Autodesk Inventor part; units mm, degrees
ref_plane "Work Plane2" through (0, 19.05, 0) normal (0, 1, 0) x (1, 0, 0)
ref_plane "YZ Plane" through (0, 0, 0) normal (1, 0, 0) x (0, 1, 0)
ref_plane "XZ Plane" through (0, 0, 0) normal (0, 1, 0) x (-1, 0, 0)
sketch "Sketch1" plane through (0, 0, 0) normal (0, 1, 0) x (-1, 0, 0)
  line L0 (-3.711, -25.8637) -> (-3.711, -32.2137)
  line L1 (-3.711, -32.2137) -> (-49.431, -32.2137)
  line L2 (-49.431, -32.2137) -> (-49.431, -25.8637)
  line L3 (-3.711, -25.8637) -> (-26.571, -6.8137)
  line L4 (-26.571, -6.8137) -> (-49.431, -25.8637)
  point P0 (0, 0)
  dimension "d0" = 6.35
  dimension "d1" = 6.35
  dimension "d2" = 45.72
  dimension "d3" = 22.86
  dimension "d4" = 22.86
  dimension "d5" = 25.4
ref_plane "Work Plane2" through (0, 19.05, 0) normal (0, 1, 0) x (1, 0, 0)
sketch "Sketch2" plane through (0, 19.05, 0) normal (0, 1, 0) x (1, 0, 0)
  line L0 (41.811, 32.2137) -> (11.331, 32.2137)
  line L1 (11.331, 32.2137) -> (11.331, 25.8637)
  line L2 (11.331, 25.8637) -> (26.571, 13.1637)
  line L3 (26.571, 13.1637) -> (41.811, 25.8637)
  line L4 (41.811, 25.8637) -> (41.811, 32.2137)
  point P0 (0, 0)
  point P1 (26.571, 6.8137)
  dimension "d8" = 6.35
  dimension "d9" = 6.35
  dimension "d10" = 15.24
  dimension "d11" = 15.24
  dimension "d12" = 30.48
  dimension "d15" = 0
loft "Loft1" add profiles "Sketch1", "Sketch2"
shell "Shell1" thickness 2.54 removed faces 1 at (26.571, 0, -23.7471)
sketch "Sketch4" plane through (26.571, 0, -6.8137) normal (0.6201737, 0.2480695, 0.7442084) x (0.7682213, 0, -0.6401844)
  line L0 (0, 0) -> (4.0652, 19.6647)
  line L1 (29.7571, 0) -> (23.9032, 19.6647)
  line L2 (29.7571, 0) -> (0, 0)
  line L3 (23.9032, 19.6647) -> (4.0652, 19.6647)
  line L4 (3.1188, 2.54) -> (6.1338, 17.1247)
  line L5 (6.1338, 17.1247) -> (22.0092, 17.1247)
  line L6 (22.0092, 17.1247) -> (26.3508, 2.54)
  line L7 (26.3508, 2.54) -> (3.1188, 2.54)
  point P0 (-24.7744, 2.9212)
  dimension "d21" = 2.54
  dimension "d22" = 2.54
  dimension "d23" = 2.54
  dimension "d24" = 2.54
extrude "Extrusion2" cut sketch "Sketch4" against normal blind 1.27 contours L4 L5 L6 L7
sketch "Sketch5" plane through (3.711, 0, -25.8637) normal (-0.6201737, 0.2480695, 0.7442084) x (0.7682213, 0, 0.6401844)
  line L0 (29.7571, 0) -> (0, 0)
  line L1 (24.1888, 19.6583) -> (4.3507, 19.6583)
  line L2 (3.4063, 2.54) -> (7.746, 17.1183)
  line L3 (7.746, 17.1183) -> (23.6246, 17.1183)
  line L4 (23.6246, 17.1183) -> (26.6383, 2.54)
  line L5 (26.6383, 2.54) -> (3.4063, 2.54)
  line L6 (0, 0) -> (5.8538, 19.6647)
  line L7 (29.7571, 0) -> (25.6919, 19.6647)
  point P0 (13.7067, -5.5182)
  point P1 (-24.7744, 2.9212)
  dimension "d27" = 2.54
  dimension "d29" = 2.54
  dimension "d32" = 2.54
  dimension "d34" = 2.54
extrude "Extrusion3" cut sketch "Sketch5" against normal blind 1.27
sketch "Sketch6" plane through (49.431, 0, -32.2137) normal (0, 0, -1) x (-1, 0, 0)
  circle A0 centre (6.985, 3.175) radius 1.5875
  circle A1 centre (22.86, 15.875) radius 1.5875
  circle A2 centre (38.735, 3.175) radius 1.5875
  line L0 (0, 0) -> (7.62, 19.05)
  line L1 (45.72, 0) -> (0, 0)
  line L2 (45.72, 0) -> (38.1, 19.05)
  line L3 (38.1, 19.05) -> (7.62, 19.05)
  point P0 (49.431, 0)
  dimension "d37" = 6.985
  dimension "d38" = 6.985
  dimension "d39" = 3.175
  dimension "d40" = 3.175
  dimension "d41" = 3.175
  dimension "d42" = 22.86
  dimension "d43" = 3.175
  dimension "d44" = 3.175
  dimension "d45" = 3.175
extrude "Extrusion4" add sketch "Sketch6" along normal blind 3.175 contours A0 | A1 | A2
chamfer "Chamfer1" distance 0.254 angle 45 3 edges at (44.0335, 3.175, -35.3887) (28.1585, 15.875, -35.3887) (12.2835, 3.175, -35.3887)
properties part number "Cow Catcher"
CAD build for the part. Positions are in the model's coordinates, mm. A direction names the side the tool comes from. Round coordinates to 2 decimals unless told otherwise and drop trailing zeros. Order: outer loops, then holes, each group sorted by start corner. A loop starts at its lowest first (then second) coordinate and runs counter-clockwise, first axis right, second up.
Q1. Slice it at A-A (z = -31.75). Write the cut outline in (x, y).
Q2. Which spindle directions (+Z, -Z, +X, -X, +Y, -Y) get a long thin tool onto all of the face, cutting with end or side? Do faces 4 (the cylindrical face through (11.956, 4.141, -33.654)), 5 (the flat face through (35.63, 8.17, -20.5)), 6 (the flat face through (11, 3, -35.389)). Say none if no direction does.
Q3. Drop flat-ended pins along their axis: pin 1 (1 mm diameter, centred on x = 38.5, y = 11, fed in from -Z); pin 2 (6 mm diameter, centred on y = 9, z = -24, fed in from -X); pin 3 (4 mm diameter, centred on x = 36.5, y = 7.5, fed in from +Z); pin 4 (11 mm diameter, centred on x = 33, z = -20, fed in from -Y). Give the stop position or say it passes through.
Q4. Two-plate mould, pull along Y, no slides. Class faces 1 (the flat face through (27, 16, -35.389)), 2 (the flat face through (43.16, 9.47, -24.63)), 3 (the flat face through (45.568, 9.658, -28.994)): pulls with the +Y half, pulls with the -Y half, needs draft (parallel to the pull), parting line crosses it, or undercut.
Q5. Wall check: L1, parallel to Y at x = 33.5, z = -28.75; L2, parallel to Z at x = 38.5, y = 4; L3, parallel to Z at x = 23, y = 8.25. Give the ranges that are in metal, low to high.
Results below:
1. outline: (3.71, 0) - (49.43, 0) - (41.81, 19.05) - (11.33, 19.05) - close
2. face 4: -Z
2. face 5: -Y
2. face 6: -Z, +X, -X, +Y, -Y
3. pin 1: stops at z = -32.21
3. pin 2: stops at x = 6.37
3. pin 3: stops at z = -17.5
3. pin 4: stops at y = 0
4. face 1: needs draft
4. face 2: undercut
4. face 3: pulls with the +Y half
5. L1: y = 16.51 to 19.05
5. L2: z = -32.21 to -29.67, -21.5 to -19.8
5. L3: z = -32.21 to -29.67, -15.95 to -14.25
